Can you work these out from the model? Positions are in its coordinate system, mm. Coordinates: 2 decimals unless noted, no trailing zeros. Order: outer loops, then holes, each group sorted by start corner. A loop starts at its lowest first (then second) coordinate and runs counter-clockwise, first axis right, second up. Notation, with made-up numbers: (-32, 79) -> (21, 79) arc R27 cw to (21, 108) -> close; hole circle Ø10 at (23, -0.5). An arc over 180 degrees is marked (long way). Use a Markdown table: item, result. Add a question column.
1. Suppose I cut it at D-D, the plane y = 14. List the corners of the cut face in (x, z) for me, then the cut area to 3 significant figures.
2. Suppose I cut it at B-B, the plane z = 1. List the corners of the cut face in (x, y) for me.
3. Suppose I cut it at A-A, the plane y = 28. List the corners of the cut face in (x, z) for me, then the cut area to 3 significant figures.
4. Suppose I cut it at C-C, the plane x = 0. List the corners of the cut face in (y, z) for me, then the cut area to 3 significant figures.
5. For pin 1 Ø12 at (x, y) = (-14, 13) entering from +Z; pin 2 Ø3 at (x, y) = (-24.25, 14) entering from -Z; pin 3 Ø1 at (y, z) = (12, 0.5) entering from -X, each with a flat end and sliding along its axis, tell me the tip position at first contact or that it passes through.
6. We'd pull the mould along X, two halves only. Please class faces 1 (the flat face through (34.036, -3.821, 0.986)), 2 (the flat face through (9, 19, 0)), 3 (the cylindrical face through (0.77, 19.985, 0.986)): pulls with the +X half, pulls with the -X half, needs draft (parallel to the pull), parting line crosses it, or undercut.
7. If I drill on line 1 along X through (y, z) = (15, 1.6); line 2 along Y through (x, z) = (25.5, 0.5); line 3 along Y through (x, z) = (0, 1.15), over which ranges is the centre line in solid material (lowest first)? Write a range as from..to.
```python
from build123d import *

# Parameters (mm, degrees)
SKETCH1_R           = 20
SKETCH1_R_2         = 2
SKETCH1_R_3         = 2.5
BOSS_EXTRUDE1_DEPTH = 2
SKETCH2_W           = 100.062981373
SKETCH2_H           = 60.5
CUT_EXTRUDE1_DEPTH  = 10
BOSS_EXTRUDE2_DEPTH = 2


with BuildPart() as part:
    # Sketch1 → Boss-Extrude1 (new body)
    with BuildSketch(Plane.XY):
        with BuildLine():
            Line((-50, -79), (50, -79))
            Line((50, -79), (31.791156311, 6.750731842))
            ThreePointArc((31.791156311, 6.750731842), (0, 32.5), (-31.791156311, 6.750731842))
            Line((-31.791156311, 6.750731842), (-50, -79))
        make_face()
        Circle(SKETCH1_R, mode=Mode.SUBTRACT)
        with Locations((0, 28)):
            Circle(SKETCH1_R_2, mode=Mode.SUBTRACT)
        with Locations((24.248711306, 14)):
            Circle(SKETCH1_R_2, mode=Mode.SUBTRACT)
        with Locations((24.248711306, -14)):
            Circle(SKETCH1_R_2, mode=Mode.SUBTRACT)
        with Locations((-24.248711306, -14)):
            Circle(SKETCH1_R_2, mode=Mode.SUBTRACT)
        with Locations((-24.248711306, 14)):
            Circle(SKETCH1_R_2, mode=Mode.SUBTRACT)
        with Locations((0, -71.5)):
            Circle(SKETCH1_R_3, mode=Mode.SUBTRACT)
        with Locations((23, -46.5)):
            Circle(SKETCH1_R_3, mode=Mode.SUBTRACT)
        with Locations((-23, -46.5)):
            Circle(SKETCH1_R_3, mode=Mode.SUBTRACT)
    extrude(amount=BOSS_EXTRUDE1_DEPTH)

    # Sketch2 → Cut-Extrude1 (cut)
    with BuildSketch(Plane(origin=(0, 0, 0), x_dir=(-1, 0, 0), z_dir=(0, 0, -1))):
        with Locations((0.031490687, -48.75)):
            Rectangle(SKETCH2_W, SKETCH2_H)
    extrude(amount=-CUT_EXTRUDE1_DEPTH, mode=Mode.SUBTRACT)

    # Sketch3 → Boss-Extrude2 (add)
    with BuildSketch(Plane.XY.offset(2)):
        with BuildLine():
            Line((-36.218763373, -14.100155361), (-37.153053746, -18.5))
            Line((-37.153053746, -18.5), (-41.739173899, -18.5))
            ThreePointArc((-41.739173899, -18.5), (-38.327081149, -17.117989866), (-36.218763373, -14.100155361))
        make_face()
    boss_extrude2 = extrude(amount=-BOSS_EXTRUDE2_DEPTH)

    # Mirror1: Boss-Extrude2 across plane
    add(boss_extrude2.mirror(Plane(origin=(0, 0, 0), x_dir=(0, 0, 1), z_dir=(1, 0, 0))))


solid = part.part
```
Worked out:
| question | item | result |
|---|---|---|
| 1 | outline | (-29.33, 0) -> (-26.25, 0) -> (-26.25, 2) -> (-29.33, 2) -> close; (-22.25, 0) -> (-14.28, 0) -> (-14.28, 2) -> (-22.25, 2) -> close; (14.28, 0) -> (22.25, 0) -> (22.25, 2) -> (14.28, 2) -> close; (26.25, 0) -> (29.33, 0) -> (29.33, 2) -> (26.25, 2) -> close |
| 1 | area | 44.2 mm² |
| 2 | outline | (-41.74, -18.5) -> (-7.6, -18.5) arc R20 cw (long way) to (7.6, -18.5) -> (41.74, -18.5) arc R6.48 cw to (36.22, -14.1) -> (31.79, 6.75) arc R32.5 ccw to (-31.79, 6.75) -> (-36.22, -14.1) arc R6.48 cw to start; hole circle Ø4 at (-24.25, -14); hole circle Ø4 at (-24.25, 14); hole circle Ø4 at (0, 28); hole circle Ø4 at (24.25, -14); hole circle Ø4 at (24.25, 14) |
| 3 | outline | (-16.5, 0) -> (-2, 0) -> (-2, 2) -> (-16.5, 2) -> close; (2, 0) -> (16.5, 0) -> (16.5, 2) -> (2, 2) -> close |
| 3 | area | 58.0 mm² |
| 4 | outline | (20, 0) -> (26, 0) -> (26, 2) -> (20, 2) -> close; (30, 0) -> (32.5, 0) -> (32.5, 2) -> (30, 2) -> close |
| 4 | area | 17.0 mm² |
| 5 | pin 1 | stops at z = 2 |
| 5 | pin 2 | passes through |
| 5 | pin 3 | stops at x = -30.4 |
| 6 | face 1 | pulls with the +X half |
| 6 | face 2 | needs draft |
| 6 | face 3 | undercut |
| 7 | line 1 | x = -28.83..-25.98, -22.52..-13.23, 13.23..22.52, 25.98..28.83 |
| 7 | line 2 | y = -18.5..-15.56, -12.44..12.44, 15.56..20.15 |
| 7 | line 3 | y = 20..26, 30..32.5 |
